Design review of the part built by this model. Coordinates are the model's own, in mm. A direction names the side the tool comes from. Round coordinates to 2 decimals unless told otherwise and drop trailing zeros. Loops run counter-clockwise (first coordinate to the right, second up) from the corner with the lowest first, then second, coordinate; pieces in that order, holes last. Notation, with made-up numbers: M 54.25,35 L 70.25,35 A8 cw 70.25,40 Z; hole C 18,10 d3. An arc over 180 degrees is marked long. Use a Markdown table: item, result.
Autodesk Inventor part; units mm, degrees
ref_plane "YZ Plane" through (0, 0, 0) normal (1, 0, 0) x (0, 1, 0)
ref_plane "XZ Plane" through (0, 0, 0) normal (0, 1, 0) x (-1, 0, 0)
ref_plane "XY Plane" through (0, 0, 0) normal (0, 0, 1) x (1, 0, 0)
sketch "Sketch1" plane through (0, 0, 0) normal (1, 0, 0) x (0, 1, 0)
  line L0 (0, 0) -> (5.5, 0)
  line L1 (5.5, 0) -> (5.5, 2)
  line L2 (5.5, 2) -> (2.5, 2)
  line L3 (2.5, 2) -> (2.5, 27)
  line L4 (2.5, 27) -> (0, 27)
  line L5 (0, 27) -> (0, 0)
  dimension "d0" = 25
  dimension "d1" = 2
  dimension "d2" = 5.5
  dimension "d3" = 2.5
revolve "Revolution1" add sketch "Sketch1" angle 360 about axis through (0, 0, 27) along (0, 0, -1)
fillet "Fillet1" radius 0.5 3 edges at (0, -5.5, 0) (0, -5.5, 2) (0, -2.5, 27)
sketch "Sketch2" plane through (0, 0, 0) normal (0, 0, -1) x (-1, 0, 0)
  circle A0 centre (0, 0) radius 5
  line L0 (1.5, -0.866) -> (0, -1.7321)
  line L1 (0, -1.7321) -> (-1.5, -0.866)
  line L2 (-1.5, -0.866) -> (-1.5, 0.866)
  line L3 (-1.5, 0.866) -> (0, 1.7321)
  line L4 (0, 1.7321) -> (1.5, 0.866)
  line L5 (1.5, 0.866) -> (1.5, -0.866)
  dimension "d6" = 3
extrude "Extrusion1" cut sketch "Sketch2" against normal blind 3 contours L0 L1 L2 L3 L4 L5
thread "Thread1"
properties part number "M5x25 low profile screw"
1. Wall thickness on line 1 along Z through (x, y) = (4, 2.75); line 2 along Z through (x, y) = (0.25, 1.25); line 3 along Y through (x, z) = (1.5, 23): over which ranges is each line inside the solid? List them lowest first. Write a range as from..to.
Check values:
| item | result |
|---|---|
| line 1 | z = 0..2 |
| line 2 | z = 3..27 |
| line 3 | y = -2..2 |
2. Take a section at B-B on z = 8.5. Give the boundary of the cut face in (x, y), and give its area (3 significant figures).
Check values:
| item | result |
|---|---|
| outline | C 0,0 d5 |
| area | 19.6 mm² |
3. Insertion check: pin 1 (5 mm diameter, centred on x = -1, z = 19.5, fed in from -Y); pin 2 (4 mm diameter, centred on x = 2, z = 20, fed in from +Y); pin 3 (0.9 mm diameter, centred on x = 0.5, y = -0.5, fed in from -Z). Each pin has a flat end and moves straight along its axis. Give the tip position at first contact, or say it passes through.
Check values:
| item | result |
|---|---|
| pin 1 | stops at y = -2.5 |
| pin 2 | stops at y = 2.5 |
| pin 3 | stops at z = 3 |
4. Machinability: for faces 1 (the face through (-0.76, -1.293, 1.479)), 2 (the face through (5.37, -1.19, 1.01)), 3 (the face through (-2, 2, 2)), which of the approach directions +Z, -Z, +X, -X, +Y, -Y give a long, thin tool a straight path to every point of the face, cutting with its end or side? Answer none if there is none.
Check values:
| item | result |
|---|---|
| face 1 | -Z |
| face 2 | +Z, -Z |
| face 3 | +Z |
5. The part is to be moulded in two halves that separate along Y. For faces 4 (the face through (0, 0, 27)), 5 (the face through (2.44, -0.54, 14.42)), 6 (the face through (0.74, -1.305, 1.479)), say which applies: pulls with the +Y half, pulls with the -Y half, needs draft (parallel to the pull), parting line crosses it, or undercut.
Check values:
| item | result |
|---|---|
| face 4 | needs draft |
| face 5 | parting line crosses it |
| face 6 | undercut |
6. Take a section at A-A on y = 0. Give the boundary of the cut face in (x, z).
Check values:
| item | result |
|---|---|
| outline | M -5.5,0.5 A0.5 ccw -5,0 L -1.5,0 L -1.5,3 L 1.5,3 L 1.5,0 L 5,0 A0.5 ccw 5.5,0.5 L 5.5,1.5 A0.5 ccw 5,2 L 2.5,2 L 2.5,26.5 A0.5 ccw 2,27 L -2,27 A0.5 ccw -2.5,26.5 L -2.5,2 L -5,2 A0.5 ccw -5.5,1.5 Z |
